from build123d import *

# Parameters (mm, degrees)
F1_DEPTH = 15
F2_R     = 7
F3_R     = 2.6
F3_R_2   = 2.1
F4_DEPTH = 25
F6_DEPTH = 2
F7_SIZE  = 5


with BuildPart() as f1:
    # F0 (on Top) → F1 (new body)
    with BuildSketch(Plane.XY):
        with BuildLine():
            Line((8.448482, -14.5), (22.25, -14.5))
            ThreePointArc((22.25, -14.5), (25.785534, -13.035534), (27.25, -9.5))
            Line((27.25, -9.5), (27.25, 9.5))
            ThreePointArc((27.25, 9.5), (25.785534, 13.035534), (22.25, 14.5))
            Line((22.25, 14.5), (8.275024, 14.5))
            Line((8.275024, 14.5), (8.275024, 22.5))
            Line((8.275024, 22.5), (1.5, 22.5))
            Line((1.5, 22.5), (1.5, 14.5))
            Line((1.5, 14.5), (1.5, 11.5))
            Line((1.5, 11.5), (19.25, 11.5))
            ThreePointArc((19.25, 11.5), (22.785534, 10.035534), (24.25, 6.5))
            Line((24.25, 6.5), (24.25, -6.5))
            ThreePointArc((24.25, -6.5), (22.785534, -10.035534), (19.25, -11.5))
            Line((19.25, -11.5), (-19.25, -11.5))
            ThreePointArc((-19.25, -11.5), (-22.785534, -10.035534), (-24.25, -6.5))
            Line((-24.25, -6.5), (-24.25, 6.5))
            ThreePointArc((-24.25, 6.5), (-22.785534, 10.035534), (-19.25, 11.5))
            Line((-19.25, 11.5), (-1.5, 11.5))
            Line((-1.5, 11.5), (-1.5, 14.5))
            Line((-1.5, 14.5), (-1.5, 22.5))
            Line((-1.5, 22.5), (-8.275024, 22.5))
            Line((-8.275024, 22.5), (-8.275024, 14.5))
            Line((-8.275024, 14.5), (-22.25, 14.5))
            ThreePointArc((-22.25, 14.5), (-25.785534, 13.035534), (-27.25, 9.5))
            Line((-27.25, 9.5), (-27.25, -9.5))
            ThreePointArc((-27.25, -9.5), (-25.785534, -13.035534), (-22.25, -14.5))
            Line((-22.25, -14.5), (-8.451518, -14.5))
            Line((-8.451518, -14.5), (-8.451518, -29.5))
            Line((-8.451518, -29.5), (-5.151518, -29.5))
            Line((-5.151518, -29.5), (-5.151518, -14.5))
            Line((-5.151518, -14.5), (-1.651518, -14.5))
            Line((-1.651518, -14.5), (-1.651518, -29.5))
            Line((-1.651518, -29.5), (1.648482, -29.5))
            Line((1.648482, -29.5), (1.648482, -14.5))
            Line((1.648482, -14.5), (5.148482, -14.5))
            Line((5.148482, -14.5), (5.148482, -29.5))
            Line((5.148482, -29.5), (8.448482, -29.5))
            Line((8.448482, -29.5), (8.448482, -14.5))
        make_face()
    extrude(amount=F1_DEPTH)

    # F2
    f2_edges = [f1.edges().sort_by_distance(p)[0] for p in [
        (-6.801518, -29.5, 15),
        (-6.801518, -29.5, 0),
        (-0.001518, -29.5, 15),
        (6.798482, -29.5, 15),
        (6.798482, -29.5, 0),
        (-0.001518, -29.5, 0),
    ]]
    fillet(f2_edges, radius=F2_R)

    # F3 (on face) → F4 (cut)
    with BuildSketch(Plane(origin=(-8.451518, 0, 0), x_dir=(0, -1, 0), z_dir=(-1, 0, 0))):
        with Locations((22.5, 7.5)):
            Circle(F3_R)
        with Locations((-18.629974, 7.5)):
            Circle(F3_R_2)
    extrude(amount=-F4_DEPTH, mode=Mode.SUBTRACT)

    # F5 (on face) → F6 (cut)
    with BuildSketch(Plane.YZ.offset(8.448482)):
        Polygon((-18.6, 5.248334), (-18.6, 9.751666), (-22.5, 12.003332), (-26.4, 9.751666), (-26.4, 5.248334), (-22.5, 2.996668), align=None)
    extrude(amount=-F6_DEPTH, mode=Mode.SUBTRACT)

    # F7
    f7_edges = [f1.edges().sort_by_distance(p)[0] for p in [
        (4.887512, 22.5, 15),
        (-4.887512, 22.5, 15),
        (4.887512, 22.5, 0),
        (-4.887512, 22.5, 0),
    ]]
    chamfer(f7_edges, length=F7_SIZE)


solid = f1.part
Source: CAD feature listing. Evaluate the final solid. Frame: model axes, mm. A direction names the side the tool comes from. Give positions to 0.01 mm unless a question says otherwise; leave off trailing zeros. Write each loop counter-clockwise with the first axis right and the second up, starting at its lowest first coordinate (ties: lowest second). Pieces come first, ordered by that corner, then holes. Notation, with made-up numbers: M 22,1 L 30,1 A22 cw 30,8 Z; hole C -30.5,47 d5. An arc over 180 degrees is marked long. Answer as a JSON object with one key per item and string values.
Q1. Cut plane B-B, the plane y = -5. Return the cut outline in (x, z).
Geometry check:
{"outline": "M -27.25,0 L -24.25,0 L -24.25,15 L -27.25,15 Z; M 24.25,0 L 27.25,0 L 27.25,15 L 24.25,15 Z"}
Q2. Ray query, line 1 along X through (y, z) = (-25, 12); line 2 along X through (y, z) = (-20, 9); line 3 along Z through (x, y) = (1, -22.5). Return the intervals inside material, ascending.
Geometry check:
{"line 1": "x = -8.45 to -5.15, -1.65 to 1.65, 5.15 to 8.45", "line 2": "x = -8.45 to -5.15, -1.65 to 1.65, 5.15 to 6.45", "line 3": "z = 0 to 4.9, 10.1 to 15"}
Q3. Cut plane A-A, the plane x = -3. Return the cut outline in (y, z).
Geometry check:
{"outline": "M -14.5,0 L -11.5,0 L -11.5,15 L -14.5,15 Z; M 11.5,0 L 17.5,0 L 22.5,5 L 22.5,10 L 17.5,15 L 11.5,15 Z; hole C 18.63,7.5 d4.2"}
Q4. Mould query, pull axis X, two halves, no side actions, for faces 1 (the face through (-5.152, -20, 6)), 2 (the face through (25.82, 13, 7.4)), 3 (the face through (0, -27.5, 12.9)). Classes: +X half, -X half, draft (parallel to the pull), parting line (faces both ways), or undercut.
Geometry check:
{"face 1": "undercut", "face 2": "+X half", "face 3": "draft"}
Q5. Contact query for flat-ended pins moving along their axis: P1, Ø8, axis at x = -13.5, z = 8.5, coming from the -Y side; P2, Ø6.5, axis at y = 18.63, z = 7.5, coming from the -X side (3 decimals); P3, Ø7, axis at y = -22.5, z = 7.5, coming from the -X side. Output: stop coordinate, or through.
Geometry check:
{"P1": "stops at y = -14.5", "P2": "stops at x = -8.275", "P3": "stops at x = -8.45"}
Q6. Cut plane D-D, the plane y = -12.5. Return the cut outline in (x, z).
Geometry check:
{"outline": "M -26.25,0 L 26.25,0 L 26.25,15 L -26.25,15 Z"}
Q7. Cut plane C-C, the plane x = 10.5. Return the cut outline in (y, z), then the cut area to 3 significant figures.
Geometry check:
{"outline": "M -14.5,0 L -11.5,0 L -11.5,15 L -14.5,15 Z; M 11.5,0 L 14.5,0 L 14.5,15 L 11.5,15 Z", "area": "90.0 mm^2"}
Q8. Access query for faces 4 (the face through (6.448, -25.2, 6.6)), 5 (the face through (-15, -14.5, 7)), 6 (the face through (1.648, -20, 6)), 7 (the face through (-22.82, 10, 7.4)), 8 (the face through (-8.275, 16, 7)). Directions: +Z, -Z, +X, -X, +Y, -Y. A direction counts if a zero-diameter tool reaches every point of the face in a straight line with its end or side. Return the directions, or none.
Geometry check:
{"face 4": "+X", "face 5": "+Z, -Z, -X, -Y", "face 6": "+Z, -Z, -Y", "face 7": "+Z, -Z", "face 8": "+Z, -Z, -X, +Y"}
